Source: CAD feature listing. Evaluate the final solid. Frame: model axes, mm. A direction names the side the tool comes from. Round coordinates to 2 decimals unless told otherwise and drop trailing zeros. Write each loop counter-clockwise with the first axis right and the second up, starting at its lowest first coordinate (ties: lowest second). Pieces come first, ordered by that corner, then holes. Notation, with made-up numbers: M 25,49.25 L 42,49.25 A12 ccw 42,53.25 Z; hole C 42,89 d6. An arc over 180 degrees is marked long. Use a Markdown table: item, result.
```python
from build123d import *

# Parameters (mm, degrees)
F1_DEPTH = 4.8
F2_R     = 2.6
F3_DEPTH = 4
F4_R     = 2.6
F5_DEPTH = 4.8
F6_R     = 2
F7_W     = 48
F7_H     = 2.3
F8_DEPTH = 25


with BuildPart() as f1:
    # F0 (on Front) → F1 (new body)
    with BuildSketch(Plane.XZ):
        with BuildLine():
            Line((-39, 0), (-39, -46))
            ThreePointArc((-39, -46), (0, -31), (39, -46))
            Line((39, -46), (39, 0))
            ThreePointArc((39, 0), (0, 9), (-39, 0))
        make_face()
    extrude(amount=-F1_DEPTH)

    # F2 (on face) → F3 (join)
    with BuildSketch(Plane.XZ):
        with Locations((-31.75, -13.3)):
            Circle(F2_R)
        with Locations((31.75, -13.3)):
            Circle(F2_R)
    extrude(amount=F3_DEPTH)

    # F4 (on face) → F5 (cut, through all)
    with BuildSketch(Plane(origin=(0, 4.8, 0), x_dir=(-1, 0, 0), z_dir=(0, 1, 0))):
        with Locations((-31.75, -20.5)):
            Circle(F4_R)
        with Locations((31.75, -20.5)):
            Circle(F4_R)
    extrude(amount=-F5_DEPTH, mode=Mode.SUBTRACT)

    # F6
    f6_edges = [f1.edges().sort_by_distance(p)[0] for p in [
        (-39, 2.4, -46),
        (39, 2.4, -46),
    ]]
    fillet(f6_edges, radius=F6_R)

    # F7 (on Top) → F8 (cut)
    with BuildSketch(Plane.XY):
        with Locations((0, 1.15)):
            Rectangle(F7_W, F7_H)
    extrude(amount=-F8_DEPTH, mode=Mode.SUBTRACT)


solid = f1.part
```
Q1. Section B-B on x = -31.75. Return loops of the section in (y, z).
Results are:
| item | result |
|---|---|
| outline | M -4,-15.9 L 0,-15.9 L 0,-17.9 L 4.8,-17.9 L 4.8,3.14 L 0,3.14 L 0,-10.7 L -4,-10.7 Z; M 0,-40.42 L 4.8,-40.42 L 4.8,-23.1 L 0,-23.1 Z |
Q2. First-contact query: pin 1 Ø4 at (x, z) = (31.75, -20.5) entering from -Y; pin 2 Ø3 at (x, z) = (-28, -37) entering from -Y; pin 3 Ø1.5 at (x, y) = (15, 0.5) entering from +Z; pin 4 Ø0.7 at (x, y) = (7.5, 0.5) entering from -Z. Flat tips, straight axial feed; report the tip coordinate or a pass-through.
Results are:
| item | result |
|---|---|
| pin 1 | through |
| pin 2 | y = 0 |
| pin 3 | z = 7.85 |
| pin 4 | z = -31.53 |
Q3. Line query: L1, parallel to Y at x = 23, z = -2; L2, parallel to Y at x = 11, z = -25.5; L3, parallel to Z at x = -31.75, y = 3.2. Output: solid intervals per line, ascending.
Results are:
| item | result |
|---|---|
| L1 | 2.3 to 4.8 |
| L2 | 0 to 4.8 |
| L3 | -40.42 to -23.1, -17.9 to 3.14 |
Q4. Section C-C on y = 1.25. Return loops of the section in (x, z), plus the area to 3 significant figures.
Results are:
| item | result |
|---|---|
| outline | M -39,-41.71 A2 ccw -35.77,-43.29 A58.2 cw 35.77,-43.29 A2 ccw 39,-41.71 L 39,0 A89 ccw -39,0 Z; hole C -31.75,-20.5 d5.2; hole M -24,-25 L 24,-25 L 24,0 L -24,0 Z; hole C 31.75,-20.5 d5.2 |
| area | 2,010 mm^2 |
Q5. Mould query, pull axis X, two halves, no side actions, for faces 3 (the flat face through (32, -4, -13)), 4 (the cylindrical face through (-31.412, 2.434, -17.922)), 5 (the cylindrical face through (0.57, 2.37, 9)). Classes: +X half, -X half, draft (parallel to the pull), parting line (faces both ways), or undercut.
Results are:
| item | result |
|---|---|
| face 3 | draft |
| face 4 | undercut |
| face 5 | parting line |
Q6. Section A-A on z = -20.5. Return loops of the section in (x, y).
Results are:
| item | result |
|---|---|
| outline | M -39,0 L -34.35,0 L -34.35,4.8 L -39,4.8 Z; M -29.15,0 L -24,0 L -24,2.3 L 24,2.3 L 24,0 L 29.15,0 L 29.15,4.8 L -29.15,4.8 Z; M 34.35,0 L 39,0 L 39,4.8 L 34.35,4.8 Z |
Q7. Reachability of faces 1 (the flat face through (0, 1, 0)), 2 (the flat face through (39, 2, -21)) from +Z, -Z, +X, -X, +Y, -Y: full face, straight path, thin tool, end or side. Return the list, or none.
Results are:
| item | result |
|---|---|
| face 1 | -Y |
| face 2 | +Z, -Z, +X, +Y, -Y |
Q8. Section D-D on z = -13.3. Return loops of the section in (x, y).
Results are:
| item | result |
|---|---|
| outline | M -39,0 L -34.35,0 L -34.35,-4 L -29.15,-4 L -29.15,0 L -24,0 L -24,2.3 L 24,2.3 L 24,0 L 29.15,0 L 29.15,-4 L 34.35,-4 L 34.35,0 L 39,0 L 39,4.8 L -39,4.8 Z |
